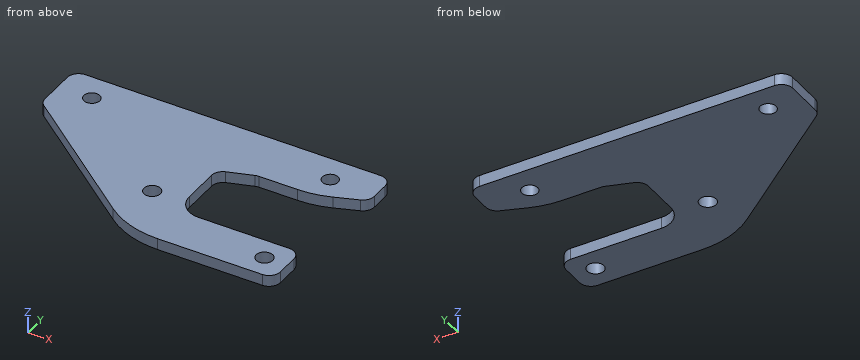
Autodesk Inventor part; units mm, degrees
ref_plane "YZ Plane" through (0, 0, 0) normal (1, 0, 0) x (0, 1, 0)
ref_plane "XZ Plane" through (0, 0, 0) normal (0, 1, 0) x (-1, 0, 0)
ref_plane "XY Plane" through (0, 0, 0) normal (0, 0, 1) x (1, 0, 0)
sketch "Sketch1" plane through (0, 0, 0) normal (0, 0, 1) x (1, 0, 0)
  line L0 (0, 0) -> (-88.9, 0)
  line L1 (0, 0) -> (0, 15.24)
  line L2 (0, 15.24) -> (-88.9, 15.24)
  line L3 (-88.9, 15.24) -> (-88.9, 0)
  line L4 (0, 0) -> (-44.45, 0)
  line L5 (-44.45, 0) -> (-44.45, -22.225)
  line L6 (0, 0) -> (-31.75, 0)
  line L7 (-31.75, 0) -> (-31.75, -22.225)
  line L8 (-44.45, -22.225) -> (-31.75, -22.225)
  line L9 (-31.75, -22.225) -> (0, -22.225)
  line L10 (0, -22.225) -> (0, -34.925)
  line L11 (0, -34.925) -> (-44.45, -34.925)
  line L12 (-44.45, -34.925) -> (-88.9, 0)
  line L13 (0, -28.575) -> (-9.525, -28.575)
  circle A0 centre (-9.525, -28.575) radius 2.3241
  line L14 (-49.0828, -48.0247) -> (-25.6113, -57.7328)
  line L15 (-44.45, 0) -> (-38.1, 0)
  line L16 (-38.1, 0) -> (-38.1, -22.225)
  line L17 (0, -28.575) -> (-3.175, -28.575)
  line L18 (-3.175, -22.225) -> (-3.175, -34.925)
  dimension "d0" = 88.9
  dimension "d1" = 15.24
  dimension "d2" = 44.45
  dimension "d3" = 22.225
  dimension "d4" = 31.75
  dimension "d5" = 12.7
  dimension "d6" = 9.525
  dimension "d7" = 4.6482
  dimension "d8" = 25.4
  dimension "d13" = 3.175
extrude "Extrusion1" add sketch "Sketch1" along normal blind 3.175
extrude "Extrusion2" cut sketch "Sketch1" along normal blind 3.175 contours L7 L8 L16 L0
extrude "Extrusion3" cut sketch "Sketch1" along normal blind 3.175 contours L9 L10 L13 L18 | L13 L10 L11 L18
fillet "Fillet1" radius 3.175 2 edges at (-3.175, -22.225, 1.5875) (-3.175, -34.925, 1.5875)
chamfer "Chamfer1" distance 3.175 distance2 9.525 1 edges at (-38.1, 0, 1.5875) measured on face at (-38.1, -7.4083, 2.1167)
fillet "Fillet2" radius 3.175 2 edges at (-38.1, -3.175, 1.5875) (-28.575, 0, 1.5875)
fillet "Fillet3" radius 6.35 1 edges at (-38.1, -22.225, 1.5875)
fillet "Fillet4" radius 25.4 1 edges at (-44.45, -34.925, 1.5875)
sketch "Sketch2" plane through (0, 0, 3.175) normal (0, 0, 1) x (1, 0, 0)
  circle A0 centre (-9.525, -28.575) radius 2.3241
  arc A1 (-51.3577, -29.4975) -> (-35.6651, -34.925) centre (-35.6651, -9.525) ccw
  line L0 (-35.6651, -34.925) -> (-6.35, -34.925)
  arc A2 (-6.35, -34.925) -> (-3.175, -31.75) centre (-6.35, -31.75) ccw
  line L1 (-3.175, -31.75) -> (-3.175, -25.4)
  arc A3 (-3.175, -25.4) -> (-6.35, -22.225) centre (-6.35, -25.4) ccw
  line L2 (-6.35, -22.225) -> (-31.75, -22.225)
  arc A4 (-38.1, -15.875) -> (-31.75, -22.225) centre (-31.75, -15.875) ccw
  line L3 (-38.1, -15.875) -> (-38.1, -5.4634)
  arc A5 (-35.929, -2.4513) -> (-38.1, -5.4634) centre (-34.925, -5.4634) ccw
  line L4 (-29.0638, -0.1629) -> (-35.929, -2.4513)
  arc A6 (-28.0598, 0) -> (-29.0638, -0.1629) centre (-28.0598, -3.175) ccw
  line L5 (-28.0598, 0) -> (0, 0)
  line L6 (0, 0) -> (0, 15.24)
  line L7 (0, 15.24) -> (-88.9, 15.24)
  line L8 (-88.9, 15.24) -> (-88.9, 0)
  line L9 (-88.9, 0) -> (-51.3577, -29.4975)
  line L10 (0, 0) -> (0, 15.24)
  line L11 (0, 7.62) -> (-12.7, 7.62)
  circle A7 centre (-12.7, 7.62) radius 2.2225
  line L12 (-88.9, 7.62) -> (-79.375, 7.62)
  circle A8 centre (-79.375, 7.62) radius 2.2225
  dimension "d23" = 4.445
  dimension "d24" = 9.525
  dimension "d25" = 4.445
  dimension "d28" = 12.7
extrude "Extrusion4" cut sketch "Sketch2" against normal blind 3.175 contours A7 | A8
chamfer "Chamfer2" distance 12.7 distance2 4.7625 1 edges at (0, 0, 1.5875) measured on face at (-18.7065, 0, 2.1167)
fillet "Fillet5" radius 25.4 1 edges at (-12.7, 0, 1.5875)
fillet "Fillet6" radius 3.175 1 edges at (0, 4.7625, 1.5875)
fillet "Fillet7" radius 3.175 1 edges at (0, 15.24, 1.5875)
fillet "Fillet8" radius 3.175 2 edges at (-88.9, 15.24, 1.5875) (-88.9, 0, 1.5875)
sketch "Sketch3" plane through (0, 0, 3.175) normal (0, 0, 1) x (1, 0, 0)
  arc A0 (-88.9, 1.5432) -> (-87.6866, -0.9534) centre (-85.725, 1.5432) ccw
  line L0 (-87.6866, -0.9534) -> (-51.3577, -29.4975)
  arc A1 (-51.3577, -29.4975) -> (-35.6651, -34.925) centre (-35.6651, -9.525) ccw
  line L1 (-35.6651, -34.925) -> (-6.35, -34.925)
  arc A2 (-6.35, -34.925) -> (-3.175, -31.75) centre (-6.35, -31.75) ccw
  line L2 (-3.175, -31.75) -> (-3.175, -25.4)
  arc A3 (-3.175, -25.4) -> (-6.35, -22.225) centre (-6.35, -25.4) ccw
  line L3 (-6.35, -22.225) -> (-31.75, -22.225)
  arc A4 (-38.1, -15.875) -> (-31.75, -22.225) centre (-31.75, -15.875) ccw
  line L4 (-38.1, -15.875) -> (-38.1, -5.4634)
  arc A5 (-35.929, -2.4513) -> (-38.1, -5.4634) centre (-34.925, -5.4634) ccw
  line L5 (-29.0638, -0.1629) -> (-35.929, -2.4513)
  arc A6 (-28.0598, 0) -> (-29.0638, -0.1629) centre (-28.0598, -3.175) ccw
  line L6 (-28.0598, 0) -> (-17.3059, 0)
  arc A7 (-17.3059, 0) -> (-8.3874, 1.6172) centre (-17.3059, 25.4) ccw
  line L7 (-2.0602, 3.9899) -> (-8.3874, 1.6172)
  arc A8 (-2.0602, 3.9899) -> (0, 6.9628) centre (-3.175, 6.9628) ccw
  line L8 (0, 6.9628) -> (0, 12.065)
  arc A9 (0, 12.065) -> (-3.175, 15.24) centre (-3.175, 12.065) ccw
  line L9 (-3.175, 15.24) -> (-85.725, 15.24)
  arc A10 (-85.725, 15.24) -> (-88.9, 12.065) centre (-85.725, 12.065) ccw
  line L10 (-88.9, 12.065) -> (-88.9, 1.5432)
  circle A11 centre (-12.7, 7.62) radius 2.2225
  circle A12 centre (-79.375, 7.62) radius 2.2225
  circle A13 centre (-9.525, -28.575) radius 2.3241
  line L11 (-9.525, -28.575) -> (-46.99, -28.575)
  line L12 (-46.99, -28.575) -> (-46.99, -18.415)
  circle A14 centre (-46.99, -18.415) radius 2.3241
  point P0 (0, 0)
  dimension "d36" = 37.465
  dimension "d37" = 10.16
  dimension "d38" = 4.6482
extrude "Extrusion5" cut sketch "Sketch3" against normal blind 25.4 contours A14
properties part number "Goal Jaw Chassis"
Could you check a few things on this model? Use its own coordinates, in mm. Round coordinates to 2 decimals unless told otherwise and drop trailing zeros. Order: outer loops, then holes, each group sorted by start corner. A loop starts at its lowest first (then second) coordinate and runs counter-clockwise, first axis right, second up.
Q1. Imagine slicing it at C-C, the plane x = -46.99. List the corners of the cut face in (y, z) for me (3 decimals).
Geometry says:
outline: (-32.261, 0) - (-20.739, 0) - (-20.739, 3.175) - (-32.261, 3.175) - close; (-16.091, 0) - (15.24, 0) - (15.24, 3.175) - (-16.091, 3.175) - close
Q2. Imagine slicing it at A-A, the plane x = -12.7. List the corners of the cut face in (y, z) for me (1 decimal), then the cut area to 3 significant figures.
Geometry says:
outline: (-34.9, 0) - (-22.2, 0) - (-22.2, 3.2) - (-34.9, 3.2) - close; (0.4, 0) - (5.4, 0) - (5.4, 3.2) - (0.4, 3.2) - close; (9.8, 0) - (15.2, 0) - (15.2, 3.2) - (9.8, 3.2) - close
area: 73.3 mm2
Q3. Imagine slicing it at B-B, the plane z = 0.5. State how many separate pieces and enclosed holes the cut face has, then the cut area to 3 significant figures.
Geometry says:
separate pieces: 1
enclosed holes: 4
area: 2,710 mm2
Q4. Imagine slicing it at D-D, the plane y = 3. List the corners of the cut face in (x, z) for me (3 decimals).
Geometry says:
outline: (-88.9, 0) - (-4.7, 0) - (-4.7, 3.175) - (-88.9, 3.175) - close
Q5. I'm going to push a flat-ended pin straight in: P1, Ø3.5, axis at x = -79.375, y = 7.62, coming from the +Z side. Where does the tip first touch, or does it pass through?
Geometry says:
P1: passes through
Q6. Please list where these lines run through material, in increasing order: probe 1 along Y at (x, z) = (-17.5, 2) (3 decimals); probe 2 along Y at (x, z) = (-12.5, 0.55) (3 decimals); probe 3 along X at (y, z) = (-29, 0.55) (3 decimals).
Geometry says:
probe 1: y = -34.925 to -22.225, 0 to 15.24
probe 2: y = -34.925 to -22.225, 0.459 to 5.407, 9.833 to 15.24
probe 3: x = -51.991 to -11.81, -7.24 to -3.175
